```python
from build123d import *

# Parameters (mm, degrees)
SKETCH1_R                      = 21.2725
BOSS_EXTRUDE1_DEPTH            = 3.175
SKETCH2_R                      = 15.875
BOSS_EXTRUDE2_DEPTH            = 9.525
F_3_16_0_1875_DIAMETER_HOLE1_D = 4.7625
F_2_56_TAPPED_HOLE3_D          = 1.778
CIRPATTERN1_COUNT              = 3
F_8_32_TAPPED_HOLE1_D          = 3.4544
F_8_32_TAPPED_HOLE1_DEPTH      = 21.2715
F_8_32_TAPPED_HOLE1_TIP        = 1.037806461


with BuildPart() as part:
    # Sketch1 → Boss-Extrude1 (new body)
    with BuildSketch(Plane.XY):
        Circle(SKETCH1_R)
    extrude(amount=BOSS_EXTRUDE1_DEPTH)

    # Sketch2 → Boss-Extrude2 (add)
    with BuildSketch(Plane.XY.offset(3.175)):
        Circle(SKETCH2_R)
    extrude(amount=BOSS_EXTRUDE2_DEPTH)

    # 3/16 (0.1875) Diameter Hole1 (through all)
    with Locations(Plane.XY.offset(12.7)):
        with Locations((0, 0)):
            Hole(F_3_16_0_1875_DIAMETER_HOLE1_D / 2)

    # #2-56 Tapped Hole3 (through all)
    with Locations(Plane.XY.offset(3.175)):
        with Locations((0, 19.05)):
            f_2_56_tapped_hole3 = Hole(F_2_56_TAPPED_HOLE3_D / 2)

    # CirPattern1: #2-56 Tapped Hole3 ×3 about axis
    cirpattern1_axis = Axis((0, 0, 0), (0, 0, 1))
    for i in range(1, CIRPATTERN1_COUNT):
        add(f_2_56_tapped_hole3.rotate(cirpattern1_axis, i * 360 / CIRPATTERN1_COUNT), mode=Mode.SUBTRACT)

    # #8-32 Tapped Hole1
    with Locations(Plane.XZ.offset(21.2725)):
        with Locations((0, 7.9248)):
            Hole(F_8_32_TAPPED_HOLE1_D / 2, depth=F_8_32_TAPPED_HOLE1_DEPTH)
            with Locations((0, 0, -(F_8_32_TAPPED_HOLE1_DEPTH + F_8_32_TAPPED_HOLE1_TIP / 2))):  # 118° drill point
                Cone(0, F_8_32_TAPPED_HOLE1_D / 2, F_8_32_TAPPED_HOLE1_TIP, mode=Mode.SUBTRACT)


solid = part.part
```
Geometry check sheet. Reference: the model listing, model coordinates, mm. A direction names the side the tool comes from. Round coordinates to 2 decimals unless told otherwise and drop trailing zeros. Loops run counter-clockwise (first coordinate to the right, second up) from the corner with the lowest first, then second, coordinate; pieces in that order, holes last. Notation, with made-up numbers: (49, 34.5) - (100, 34.5) arc R24 ccw to (100, 47.5) - close; hole circle Ø11 at (88, 5.25). An arc over 180 degrees is marked (long way). Write item = value, one per line. Start each with the question number.
1. Set-up check for faces 1 (the face through (-3.441, -15.497, 7.871)), 2 (the face through (0, -4, 0)): record each of +Z, -Z, +X, -X, +Y, -Y from which the full face is reachable in a straight line by a thin tool's end or side.
2. Section check C-C on y = -12. Enter the section's corners in (x, z) (3 decimals), then the cut area to 3 significant figures.
3. Section check B-B on y = 0. Enter the section's corners in (x, z) (1 decimal), then the cut area to 3 significant figures.
4. Depth check by flat-ended pin: pin 1 (6 mm diameter, centred on x = 3, z = 10.5, fed in from +Y) (3 decimals); pin 2 (1.1 mm diameter, centred on x = -16.5, y = -9.52, fed in from +Z); pin 3 (1 mm diameter, centred on x = -10.5, y = 14, fed in from -Z); pin 4 (4 mm diameter, centred on y = 6.5, z = 6, fed in from -X). Enter the tip coordinate at first touch or a pass-through.
5. Mould release check, pull along Y, two halves, no side actions. Record for faces 3 (the face through (-16.881, -12.944, 1.565)), 4 (the face through (0.655, 19.651, 1.565)), 5 (the face through (-1.595, -8.659, 7.263)): released by +Y, released by -Y, zero draft, split by the parting line, or undercut.
6. Thickness scan on line 1 (Y direction, x = 0, z = 0.75); line 2 (Z direction, x = 0, y = -6.75); line 3 (Y direction, x = -0.5, z = 3). Record the ranges inside material, lowest first.
7. Section check A-A on x = 0. Enter the section's corners in (y, z) (1 decimal).
Working result:
q1.face_1 = +Z
q1.face_2 = -Z, +X, -X, +Y, -Y
q2.outline = (-17.565, 0) - (17.565, 0) - (17.565, 3.175) - (10.393, 3.175) - (10.393, 12.7) - (-10.393, 12.7) - (-10.393, 3.175) - (-17.565, 3.175) - close; hole circle Ø3.454 at (0, 7.925)
q2.area = 300 mm^2
q3.outline = (-21.3, 0) - (-2.4, 0) - (-2.4, 12.7) - (-15.9, 12.7) - (-15.9, 3.2) - (-21.3, 3.2) - close; (2.4, 0) - (21.3, 0) - (21.3, 3.2) - (15.9, 3.2) - (15.9, 12.7) - (2.4, 12.7) - close
q3.area = 377 mm^2
q4.pin_1 = 15.875
q4.pin_2 = through
q4.pin_3 = 0
q4.pin_4 = -15.22
q5.face_3 = split by the parting line
q5.face_4 = undercut
q5.face_5 = zero draft
q6.line_1 = -21.27 to -2.38, 2.38 to 18.16, 19.94 to 21.27
q6.line_2 = 0 to 6.2, 9.65 to 12.7
q6.line_3 = -21.27 to -2.33, 2.33 to 18.31, 19.79 to 21.27
q7.outline = (-21.3, 0) - (-2.4, 0) - (-2.4, 6.2) - (-15.9, 6.2) - (-15.9, 3.2) - (-21.3, 3.2) - close; (-15.9, 9.7) - (-2.4, 9.7) - (-2.4, 12.7) - (-15.9, 12.7) - close; (2.4, 0) - (18.2, 0) - (18.2, 3.2) - (15.9, 3.2) - (15.9, 12.7) - (2.4, 12.7) - close; (19.9, 0) - (21.3, 0) - (21.3, 3.2) - (19.9, 3.2) - close
